Check sheet for the drawn part. Datum: minimum x, y, z corner. Units: mm. A direction names the side the tool comes from. Round coordinates to 2 decimals unless told otherwise and drop trailing zeros. Order: outer loops, then holes, each group sorted by start corner. A loop starts at its lowest first (then second) coordinate and runs counter-clockwise, first axis right, second up.
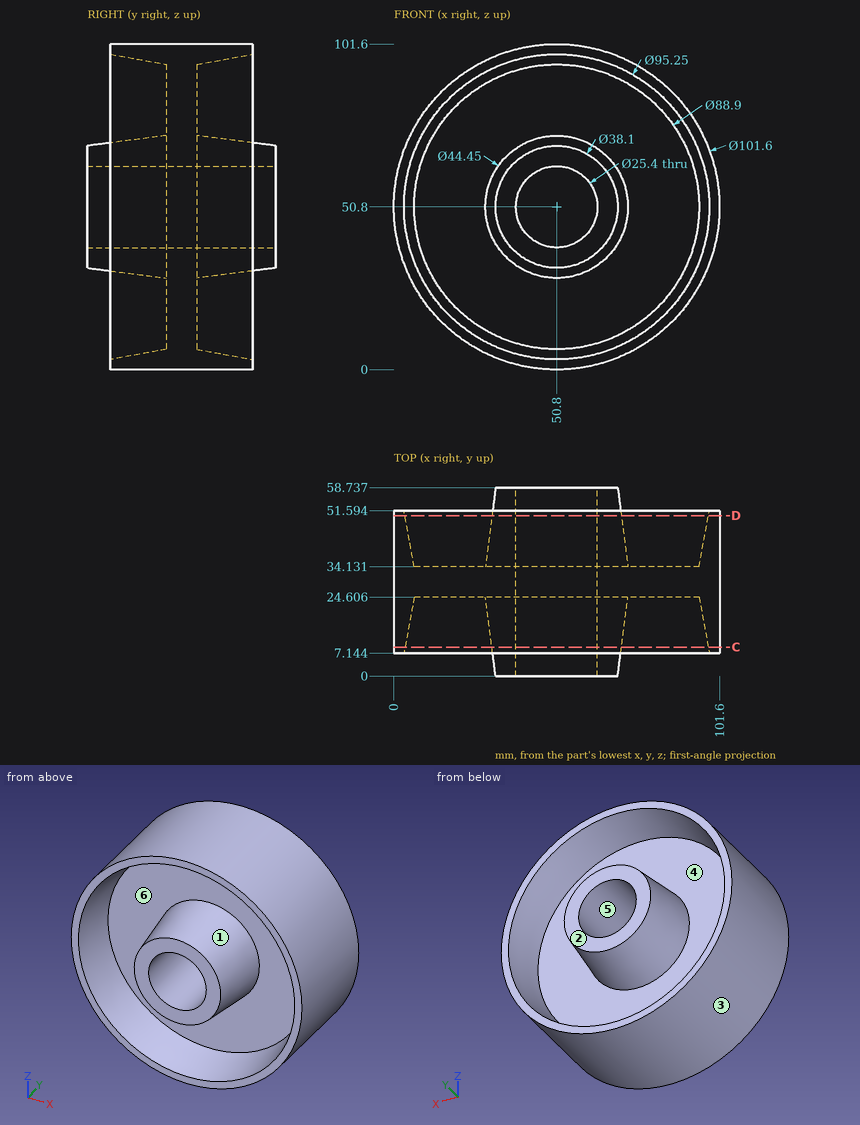
1) Sectioned sample at D-D on y = 50. Record the cut outline in (x, z) (1 decimal), and give its area (3 significant figures).
2) Gauge pin test, flat ends, axial feed: pin 1 (5 mm diameter, centred on x = 17.5, y = 7, fed in from +Z) (1 decimal); pin 2 (12 mm diameter, centred on x = 75, y = 7, fed in from +Z); pin 3 (1 mm diameter, centred on x = 43, z = 75.5, fed in from -Y). Record the tip position at first contact, or that the pin passes through.
3) Draft check along X on the marked faces 1, 2 and 3. Enter one of: pulls with the +X half, pulls with the -X half, needs draft (parallel to the pull), parting line crosses it, or undercut.
4) Scan lines: line 1 (X direction, y = 25, z = 50.8); line 2 (Z direction, x = 50, y = 16) (1 decimal); line 3 (Z direction, x = 32.5, y = 18.5) (1 decimal). Record each from-to range of solid material in increasing order.
5) Set-up check for the marked faces 4, 5 and 6: record each of +Z, -Z, +X, -X, +Y, -Y from which the full face is reachable in a straight line by a thin tool's end or side.
6) Sectioned sample at C-C on y = 9. Record the cut outline in (x, z) (1 decimal), and give its area (3 significant figures).
Values found:
1. outline: circle Ø101.6 at (50.8, 50.8); circle Ø40.4 at (50.8, 50.8); hole circle Ø94.7 at (50.8, 50.8); hole circle Ø25.4 at (50.8, 50.8)
1. area: 1,840 mm2
2. pin 1: stops at z = 91.2
2. pin 2: stops at z = 98.23
2. pin 3: stops at y = 24.61
3. face 1: undercut
3. face 2: needs draft
3. face 3: parting line crosses it
4. line 1: x = 0 to 38.1, 63.5 to 101.6
4. line 2: z = 0 to 4.8, 29.7 to 38.1, 63.5 to 71.9, 96.8 to 101.6
4. line 3: z = 3.4 to 9.1, 39.6 to 62, 92.5 to 98.2
5. face 4: +Y
5. face 5: +Y, -Y
5. face 6: -Y
6. outline: circle Ø101.6 at (50.8, 50.8); circle Ø40.4 at (50.8, 50.8); hole circle Ø94.6 at (50.8, 50.8); hole circle Ø25.4 at (50.8, 50.8)
6. area: 1,860 mm2
